from build123d import *

# Parameters (mm, degrees)
BLANKSKE_W          = 500
BLANKSKE_H          = 24
BLANK_DEPTH         = 40
TOOTHCUTSIM_DEPTH   = 503.171285519
TEETHCUTS_COUNT     = 21
TEETHCUTS_PITCH     = 25.1327412
SKETCH1_W           = 800
SKETCH1_H           = 40
BOSS_EXTRUDE1_DEPTH = 30
SKETCH2_W           = 40
SKETCH2_H           = 30
CUT_EXTRUDE1_DEPTH  = 300
SKETCH3_W           = 500.753658957
SKETCH3_H           = 40
CUT_EXTRUDE3_DEPTH  = 10


with BuildPart() as part:
    # BlankSke → Blank (new body)
    with BuildSketch(Plane.XY):
        with Locations((250, 12)):
            Rectangle(BLANKSKE_W, BLANKSKE_H)
    extrude(amount=-BLANK_DEPTH)

    # TooCutSkeSim → ToothCutSim (cut, through all)
    with BuildSketch(Plane.XY):
        Polygon((3.408482957, 6), (-3.408482957, 6), (-9.969192018, 24.0254), (9.969192018, 24.0254), align=None)
    toothcutsim = extrude(amount=-TOOTHCUTSIM_DEPTH, mode=Mode.SUBTRACT)

    # TeethCuts: ToothCutSim ×21
    with Locations(*[(i * TEETHCUTS_PITCH, 0, 0) for i in range(1, TEETHCUTS_COUNT)]):
        add(toothcutsim, mode=Mode.SUBTRACT)

    # Sketch1 → Boss-Extrude1 (add)
    with BuildSketch(Plane.XZ):
        with Locations((99.246341043, -20)):
            Rectangle(SKETCH1_W, SKETCH1_H)
    extrude(amount=BOSS_EXTRUDE1_DEPTH)

    # Sketch2 → Cut-Extrude1 (cut)
    with BuildSketch(Plane.ZY.offset(300.753658957)):
        with Locations((-20, -15)):
            Rectangle(SKETCH2_W, SKETCH2_H)
    extrude(amount=-CUT_EXTRUDE1_DEPTH, mode=Mode.SUBTRACT)

    # Sketch3 → Cut-Extrude3 (cut)
    with BuildSketch(Plane.XZ.offset(30)):
        with Locations((249.623170522, -20)):
            Rectangle(SKETCH3_W, SKETCH3_H)
    extrude(amount=-CUT_EXTRUDE3_DEPTH, mode=Mode.SUBTRACT)


solid = part.part
Design review of the part built by this model. Coordinates are the model's own, in mm. A direction names the side the tool comes from. Give positions to 0.01 mm unless a question says otherwise; leave off trailing zeros. Answer as a JSON object with one key per item and string values.
Item 1: Wall thickness on line 1 along X through (y, z) = (-8, -37.5); line 2 along Y through (x, z) = (223.5, -22); line 3 along X through (y, z) = (1, -10.5): over which ranges is each line inside the solid? List them lowest first.
Output values:
{"line 1": "x = -0.75 to 499.25", "line 2": "y = -20 to 6", "line 3": "x = 0 to 500"}
Item 2: For P1, Ø5, axis at y = -6, z = -7, coming from the +X side; P2, Ø5.5, axis at x = 75, z = -27, coming from the +Y side, all flat-tipped, find the tip position at first contact; note any pin that passes through.
Output values:
{"P1": "stops at x = 499.25", "P2": "stops at y = 6"}
Item 3: Machinability: for faces 4 (the face through (333.456, 15.126, -19.72)), 5 (the face through (246, -3, -40)), which of the approach directions +Z, -Z, +X, -X, +Y, -Y give a long, thin tool a straight path to every point of the face, cutting with its end or side? Answer none if there is none.
Output values:
{"face 4": "+Z, -Z, +Y", "face 5": "-Z, +X, -X, +Y, -Y"}
Item 4: Mouldability with a two-part tool opening along X and no side actions: class faces 1 (the face through (-0.754, -10, -20)), 2 (the face through (182.66, 15.13, -19.72)), 3 (the face through (496.02, 14.87, -19.72)) as pulls with the +X half, pulls with the -X half, needs draft (parallel to the pull), parting line crosses it, or undercut.
Output values:
{"face 1": "pulls with the -X half", "face 2": "undercut", "face 3": "pulls with the +X half"}
Item 5: We need section A-A (y = 13.5). Count the separate pieces of the cut face and the enclosed holes in it, and give its area (3 significant figures).
Output values:
{"separate pieces": "20", "enclosed holes": "0", "area": "10,300 mm2"}
